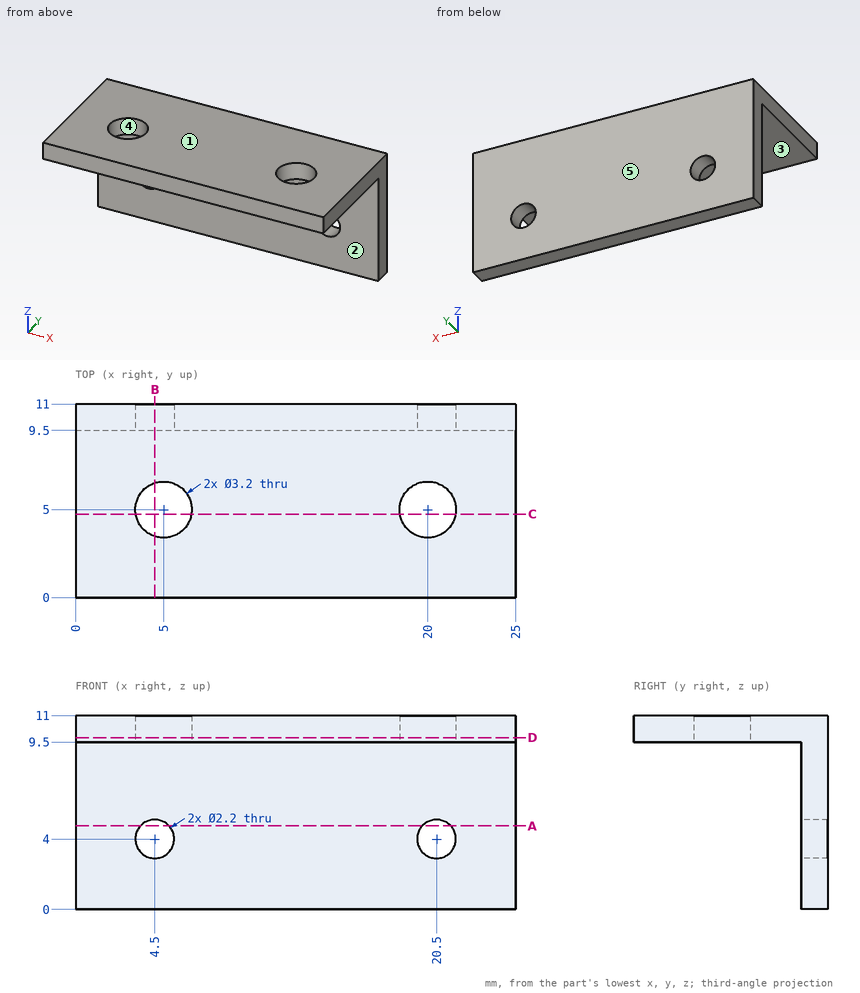
Geometry: see drawing. Coordinates: mm, zero at the bounding-box minimum. A direction names the side the tool comes from. Coordinates: 2 decimals unless noted, no trailing zeros. Loops run counter-clockwise (first coordinate to the right, second up) from the corner with the lowest first, then second, coordinate; pieces in that order, holes last.
Q1. Cut plane C-C (y = 4.75). Output: boundary loops of the cut face in (x, z), then the cut area to 3 significant figures.
Q2. Material intervals for line 1 (X direction, y = 5, z = 10.6); line 2 (X direction, y = 9.85, z = 4); line 3 (Z direction, x = 20.5, y = 10.4), sorted ascending.
Q3. Cut plane D-D (z = 9.75). Output: boundary loops of the cut face in (x, y), then the cut area to 3 significant figures.
Q4. Set-up query: the marked faces 1 and 2. Return all of +Z, -Z, +X, -X, +Y, -Y with unobstructed straight access to the full face (end or side cutting, diameter ignored); none if empty.
Q5. Contact query for flat-ended pins moving along their axis: pin 1 (2 mm diameter, centred on x = 4.5, z = 4, fed in from -Y); pin 2 (1 mm diameter, centred on x = 13, z = 4, fed in from -Y); pin 3 (5 mm diameter, centred on x = 20, y = 5, fed in from -Z). Output: stop coordinate, or through.
Q6. Cut plane A-A (z = 4.75). Output: boundary loops of the cut face in (x, y), then the cut area to 3 significant figures.
Q7. Cut plane B-B (x = 4.5). Output: boundary loops of the cut face in (y, z).
Q8. Draft query along Y for the marked faces 3, 4 and 5. Return one class per face: +Y half, -Y half, draft (parallel to the pull), parting line (faces both ways), or undercut.
Working result:
1. outline: (0, 9.5) - (3.42, 9.5) - (3.42, 11) - (0, 11) - close; (6.58, 9.5) - (18.42, 9.5) - (18.42, 11) - (6.58, 11) - close; (21.58, 9.5) - (25, 9.5) - (25, 11) - (21.58, 11) - close
1. area: 28.0 mm2
2. line 1: x = 0 to 3.4, 6.6 to 18.4, 21.6 to 25
2. line 2: x = 0 to 3.4, 5.6 to 19.4, 21.6 to 25
2. line 3: z = 0 to 2.9, 5.1 to 11
3. outline: (0, 0) - (25, 0) - (25, 11) - (0, 11) - close; hole circle Ø3.2 at (5, 5); hole circle Ø3.2 at (20, 5)
3. area: 259 mm2
4. face 1: +Z, +X, -X, +Y, -Y
4. face 2: -Z, +X, -X, -Y
5. pin 1: passes through
5. pin 2: stops at y = 9.5
5. pin 3: stops at z = 9.5
6. outline: (0, 9.5) - (3.7, 9.5) - (3.7, 11) - (0, 11) - close; (5.3, 9.5) - (19.7, 9.5) - (19.7, 11) - (5.3, 11) - close; (21.3, 9.5) - (25, 9.5) - (25, 11) - (21.3, 11) - close
6. area: 32.7 mm2
7. outline: (0, 9.5) - (3.48, 9.5) - (3.48, 11) - (0, 11) - close; (6.52, 9.5) - (9.5, 9.5) - (9.5, 5.1) - (11, 5.1) - (11, 11) - (6.52, 11) - close; (9.5, 0) - (11, 0) - (11, 2.9) - (9.5, 2.9) - close
8. face 3: draft
8. face 4: undercut
8. face 5: +Y half
